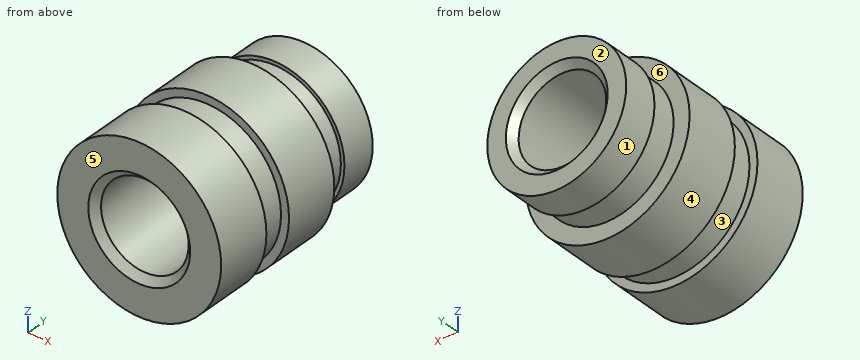
Autodesk Inventor part; units mm, degrees
ref_plane "YZ Plane" through (0, 0, 0) normal (1, 0, 0) x (0, 1, 0)
ref_plane "XZ Plane" through (0, 0, 0) normal (0, 1, 0) x (-1, 0, 0)
ref_plane "XY Plane" through (0, 0, 0) normal (0, 0, 1) x (1, 0, 0)
sketch "Sketch1" plane through (0, 0, 0) normal (0, 1, 0) x (-1, 0, 0)
  circle A0 centre (0, 0) radius 2.3
  dimension "d0" = 4.6
extrude "Extrusion1" add sketch "Sketch1" along normal blind 1.6
sketch "Sketch2" plane through (0, 1.6, 0) normal (0, 1, 0) x (1, 0, 0)
  circle A0 centre (0, 0) radius 2.075
  dimension "d3" = 4.15
extrude "Extrusion2" add sketch "Sketch2" along normal blind 0.8
sketch "Sketch3" plane through (0, 2.4, 0) normal (0, 1, 0) x (1, 0, 0)
  circle A0 centre (0, 0) radius 2.3
extrude "Extrusion3" add sketch "Sketch3" along normal blind 1.6
sketch "Sketch4" plane through (0, 4, 0) normal (0, 1, 0) x (1, 0, 0)
  circle A0 centre (0, 0) radius 1.85
  dimension "d8" = 3.7
extrude "Extrusion4" add sketch "Sketch4" along normal blind 0.8
sketch "Sketch5" plane through (0, 4.8, 0) normal (0, 1, 0) x (1, 0, 0)
  circle A0 centre (0, 0) radius 1.95
  dimension "d11" = 3.9
extrude "Extrusion5" add sketch "Sketch5" along normal blind 1
hole "Hole1" at (0, 0, 0) direction (0, 1, 0) diameter 2.459 end through all
chamfer "Chamfer1" distance 0.2 angle 45 2 edges at (0, 0, 1.2295) (0, 5.8, 1.2295)
properties part number "COTS_BOSSARD_1386867_M3_Insert"
The model under review builds one solid part; all positions refer to its coordinate system, in mm. Face numbers are marked on the shaded views. A direction names the side the tool comes from. Round coordinates to 2 decimals unless told otherwise and drop trailing zeros. Write each loop counter-clockwise with the first axis right and the second up, starting at its lowest first coordinate (ties: lowest second). Pieces come first, ordered by that corner, then holes. Notation, with made-up numbers: (-29, -16.5) - (15, -16.5) arc R14 ccw to (15, 1.5) - close; hole circle Ø7 at (19.5, -3). An arc over 180 degrees is marked (long way). One line per item, written item: value. Start each with the question number.
1. To check wall thickness, follow L1, parallel to Z at x = 0, y = 1.5; L2, parallel to Y at x = 0.75, z = -2.1; L3, parallel to X at y = 4.25, z = 0. State the ranges of each line that lie inside material, in increasing order. Write a range as from..to.
2. Machinability: for the marked faces 1, 2 and 3, which of the approach directions +Z, -Z, +X, -X, +Y, -Y give a long, thin tool a straight path to every point of the face, cutting with its end or side? Answer none if there is none.
3. Consider section C-C on y = 2.65. Write out the cut boundary in (x, z).
4. Consider section D-D on x = 1.5. Write out the cut boundary in (y, z).
5. The part is to be moulded in two halves that separate along Y. For the marked faces 4, 5 and 6, say which applies: released by +Y, released by -Y, zero draft, split by the parting line, or undercut.
6. Clearance check with flat-ended pins moving along their axes: P1, Ø2, axis at x = -1.5, y = 3, coming from the -Z side (3 decimals); P2, Ø1.5, axis at y = 5, z = -1.5, coming from the -X side. State where each tip first meets the part, or that it passes through.
Checks:
1. L1: z = -2.3..-1.23, 1.23..2.3
1. L2: y = 0..1.6, 2.4..4
1. L3: x = -1.85..-1.23, 1.23..1.85
2. face 1: +Y
2. face 2: +Z, -Z, +X, -X, +Y
2. face 3: none
3. outline: circle Ø4.6 at (0, 0); hole circle Ø2.46 at (0, 0)
4. outline: (0, -1.74) - (1.6, -1.74) - (1.6, -1.43) - (2.4, -1.43) - (2.4, -1.74) - (4, -1.74) - (4, -1.08) - (4.8, -1.08) - (4.8, -1.25) - (5.8, -1.25) - (5.8, 1.25) - (4.8, 1.25) - (4.8, 1.08) - (4, 1.08) - (4, 1.74) - (2.4, 1.74) - (2.4, 1.43) - (1.6, 1.43) - (1.6, 1.74) - (0, 1.74) - close
5. face 4: zero draft
5. face 5: released by -Y
5. face 6: undercut
6. P1: stops at z = -2.245
6. P2: stops at x = -1.8
